The listing builds one solid part. Answer for the finished solid, in the listing's coordinates (mm). Coordinates: 2 decimals unless noted, no trailing zeros. Answer in a Markdown table with one row per item. Add a question column.
from build123d import *

# Parameters (mm, degrees)
SKETCH1_W           = 609.6
SKETCH1_H           = 101.6
BOSS_EXTRUDE1_DEPTH = 3.175
SKETCH2_R           = 2.38125
CUT_EXTRUDE1_DEPTH  = 310.020647571
CUT_EXTRUDE2_DEPTH  = 310.020647571
FILLET1_R           = 5.08
SKETCH4_W           = 50.8
SKETCH4_H           = 50.8
CUT_EXTRUDE3_DEPTH  = 310.020647571


with BuildPart() as part:
    # Sketch1 → Boss-Extrude1 (new body)
    with BuildSketch(Plane.XY):
        Rectangle(SKETCH1_W, SKETCH1_H)
    extrude(amount=BOSS_EXTRUDE1_DEPTH)

    # Sketch2 → Cut-Extrude1 (cut, through all)
    with BuildSketch(Plane.XY.offset(3.175)):
        with Locations((-292.1, 38.1)):
            Circle(SKETCH2_R)
        with Locations((-292.1, -38.1)):
            Circle(SKETCH2_R)
        with Locations((-266.7, 38.1)):
            Circle(SKETCH2_R)
        with Locations((-266.7, -38.1)):
            Circle(SKETCH2_R)
        with Locations((-292.1, -19.05)):
            Circle(SKETCH2_R)
        with Locations((-266.7, -19.05)):
            Circle(SKETCH2_R)
        with Locations(Location((266.7, -19.05, 0), (0, 0, 180))):
            Circle(SKETCH2_R)
        with Locations(Location((292.1, -19.05, 0), (0, 0, 180))):
            Circle(SKETCH2_R)
        with Locations(Location((266.7, -38.1, 0), (0, 0, 180))):
            Circle(SKETCH2_R)
        with Locations(Location((266.7, 38.1, 0), (0, 0, 180))):
            Circle(SKETCH2_R)
        with Locations(Location((292.1, -38.1, 0), (0, 0, 180))):
            Circle(SKETCH2_R)
        with Locations(Location((292.1, 38.1, 0), (0, 0, 180))):
            Circle(SKETCH2_R)
    extrude(amount=-CUT_EXTRUDE1_DEPTH, mode=Mode.SUBTRACT)

    # Sketch3 → Cut-Extrude2 (cut, through all)
    with BuildSketch(Plane.XY.offset(3.175)):
        Polygon((-176.29121265, -25.4), (-205.620606325, 25.4), (-234.95, -25.4), align=None)
        Polygon((-164.55945518, -25.4), (-135.230061506, 25.4), (-193.888848855, 25.4), align=None)
        Polygon((-92.583618834, -25.4), (-121.913012509, 25.4), (-151.242406183, -25.4), align=None)
        Polygon((-80.851861364, -25.4), (-51.522467689, 25.4), (-110.181255039, 25.4), align=None)
        Polygon((-8.876025017, -25.4), (-38.205418692, 25.4), (-67.534812367, -25.4), align=None)
        Polygon((2.855732453, -25.4), (32.185126128, 25.4), (-26.473661222, 25.4), align=None)
        Polygon((74.8315688, -25.4), (45.502175125, 25.4), (16.17278145, -25.4), align=None)
        Polygon((86.563326269, -25.4), (115.892719944, 25.4), (57.233932595, 25.4), align=None)
        Polygon((158.539162616, -25.4), (129.209768941, 25.4), (99.880375267, -25.4), align=None)
        Polygon((170.270920086, -25.4), (199.600313761, 25.4), (140.941526411, 25.4), align=None)
    extrude(amount=-CUT_EXTRUDE2_DEPTH, mode=Mode.SUBTRACT)

    # Fillet1
    fillet1_edges = [part.edges().sort_by_distance(p)[0] for p in [
        (74.8315688, -25.4, 1.5875),
        (16.17278145, -25.4, 1.5875),
        (45.502175125, 25.4, 1.5875),
        (2.855732453, -25.4, 1.5875),
        (-26.473661222, 25.4, 1.5875),
        (32.185126128, 25.4, 1.5875),
        (158.539162616, -25.4, 1.5875),
        (99.880375267, -25.4, 1.5875),
        (129.209768941, 25.4, 1.5875),
        (86.563326269, -25.4, 1.5875),
        (57.233932595, 25.4, 1.5875),
        (115.892719944, 25.4, 1.5875),
        (-92.583618834, -25.4, 1.5875),
        (-151.242406183, -25.4, 1.5875),
        (-121.913012509, 25.4, 1.5875),
        (-164.55945518, -25.4, 1.5875),
        (-193.888848855, 25.4, 1.5875),
        (-135.230061506, 25.4, 1.5875),
        (-8.876025017, -25.4, 1.5875),
        (-67.534812367, -25.4, 1.5875),
        (-38.205418692, 25.4, 1.5875),
        (-80.851861364, -25.4, 1.5875),
        (-110.181255039, 25.4, 1.5875),
        (-51.522467689, 25.4, 1.5875),
        (170.270920086, -25.4, 1.5875),
        (140.941526411, 25.4, 1.5875),
        (199.600313761, 25.4, 1.5875),
        (-176.29121265, -25.4, 1.5875),
        (-234.95, -25.4, 1.5875),
        (-205.620606325, 25.4, 1.5875),
    ]]
    fillet(fillet1_edges, radius=FILLET1_R)

    # Sketch4 → Cut-Extrude3 (cut, through all)
    with BuildSketch(Plane.XY.offset(3.175)):
        with Locations((-279.4, 0)):
            Rectangle(SKETCH4_W, SKETCH4_H)
        with Locations((279.4, 0)):
            Rectangle(SKETCH4_W, SKETCH4_H)
    extrude(amount=-CUT_EXTRUDE3_DEPTH, mode=Mode.SUBTRACT)


solid = part.part
(1) A cutting plane is placed at A-A (z = 2.5). State how many separate pieces and enclosed holes the cut face has, plus the area to 3 significant figures.
(2) Straight lines are drawn through the part: line 1 (Y direction, x = -266.7, z = 2); line 2 (X direction, y = 39, z = 1.7); line 3 (Y direction, x = 142, z = 0.75). For each, find the intervals that lie inside material, in ascending order.
(3) The mould has two halves that part along Y. Classify faces 1 (the face through (-4, -22, 0)), 2 (the face through (30.98, 0.25, 1.61)), 3 (the face through (-220.14, 0.25, 1.61)): released by +Y, released by -Y, zero draft, split by the parting line, or undercut.
(4) Each of these flat-tipped pins is pushed along its axis until it touches: pin 1 (10 mm diameter, centred on x = -16, y = -16, fed in from +Z) (3 decimals); pin 2 (1 mm diameter, centred on y = 0.5, z = 2, fed in from -X). Where does it stop, or does it pass through?
Solved:
| question | item | result |
|---|---|---|
| 1 | separate pieces | 1 |
| 1 | enclosed holes | 18 |
| 1 | area | 42,300 mm² |
| 2 | line 1 | y = -50.8 to -40.48, -35.72 to -25.4, 25.4 to 35.72, 40.48 to 50.8 |
| 2 | line 2 | x = -304.8 to -294.3, -289.9 to -268.9, -264.5 to 264.5, 268.9 to 289.9, 294.3 to 304.8 |
| 2 | line 3 | y = -50.8 to -25.4, 3.25 to 50.8 |
| 3 | face 1 | zero draft |
| 3 | face 2 | undercut |
| 3 | face 3 | undercut |
| 4 | pin 1 | stops at z = 3.175 |
| 4 | pin 2 | stops at x = -254 |
